Model file for the job. Use its own axes, mm. A direction names the side the tool comes from. Coordinates: 2 decimals unless noted, no trailing zeros. Order: outer loops, then holes, each group sorted by start corner. A loop starts at its lowest first (then second) coordinate and runs counter-clockwise, first axis right, second up.
from build123d import *

# Parameters (mm, degrees)
BOSS_EXTRUDE1_DEPTH = 52
SKETCH4_W           = 4
SKETCH4_H           = 10
CUT_EXTRUDE1_DEPTH  = 6
SKETCH5_W           = 4
SKETCH5_H           = 10
CUT_EXTRUDE2_DEPTH  = 6
CUT_EXTRUDE3_DEPTH  = 3
CUT_EXTRUDE4_DEPTH  = 3
SKETCH8_R           = 1
CUT_EXTRUDE5_DEPTH  = 10
SKETCH9_R           = 1
CUT_EXTRUDE6_DEPTH  = 10


with BuildPart() as part:
    # Sketch1 → Boss-Extrude1 (new body)
    with BuildSketch(Plane.XY):
        Polygon((-37.100108605, 13.346711561), (-47.100108605, 3.346711561), (-32.100108605, 3.346711561), (-32.100108605, 13.346711561), align=None)
    extrude(amount=BOSS_EXTRUDE1_DEPTH)

    # Sketch4 → Cut-Extrude1 (cut)
    with BuildSketch(Plane.XY.offset(52)):
        with Locations((-34.100108605, 8.346711561)):
            Rectangle(SKETCH4_W, SKETCH4_H)
    extrude(amount=-CUT_EXTRUDE1_DEPTH, mode=Mode.SUBTRACT)

    # Sketch5 → Cut-Extrude2 (cut)
    with BuildSketch(Plane(origin=(0, 0, 0), x_dir=(-1, 0, 0), z_dir=(0, 0, -1))):
        with Locations((34.100108605, 8.346711561)):
            Rectangle(SKETCH5_W, SKETCH5_H)
    extrude(amount=-CUT_EXTRUDE2_DEPTH, mode=Mode.SUBTRACT)

    # Sketch6 → Cut-Extrude3 (cut)
    with BuildSketch(Plane.XY.offset(52)):
        Polygon((-47.100108605, 3.346711561), (-37.100108605, 13.346711561), (-36.100108605, 13.346711561), (-36.100108605, 3.346711561), align=None)
    extrude(amount=-CUT_EXTRUDE3_DEPTH, mode=Mode.SUBTRACT)

    # Sketch7 → Cut-Extrude4 (cut)
    with BuildSketch(Plane(origin=(0, 0, 0), x_dir=(-1, 0, 0), z_dir=(0, 0, -1))):
        Polygon((47.100108605, 3.346711561), (37.100108605, 13.346711561), (36.100108605, 13.346711561), (36.100108605, 3.346711561), align=None)
    extrude(amount=-CUT_EXTRUDE4_DEPTH, mode=Mode.SUBTRACT)

    # Sketch8 → Cut-Extrude5 (cut)
    with BuildSketch(Plane(origin=(0, 0, 6), x_dir=(-1, 0, 0), z_dir=(0, 0, -1))):
        with Locations((34.100108605, 8.346711561)):
            Circle(SKETCH8_R)
    extrude(amount=-CUT_EXTRUDE5_DEPTH, mode=Mode.SUBTRACT)

    # Sketch9 → Cut-Extrude6 (cut)
    with BuildSketch(Plane.XY.offset(46)):
        with Locations((-34.100108605, 8.346711561)):
            Circle(SKETCH9_R)
    extrude(amount=-CUT_EXTRUDE6_DEPTH, mode=Mode.SUBTRACT)


solid = part.part
Q1. Cut at A-A, the plane y = 12.5. List the corners of the cut face in (x, z), plus the area to 3 significant figures.
Established:
outline: (-37.95, 3) - (-36.1, 3) - (-36.1, 6) - (-32.1, 6) - (-32.1, 46) - (-36.1, 46) - (-36.1, 49) - (-37.95, 49) - close
area: 245 mm2
Q2. Probe line 1 (Z direction, x = -36, y = 9); line 2 (X direction, y = 8, z = 14); line 3 (Y direction, x = -42.75, z = 15.5). List the from-to ranges inside material, lowest first.
Established:
line 1: z = 6 to 46
line 2: x = -42.45 to -35.04, -33.16 to -32.1
line 3: y = 3.35 to 7.7
Q3. Drop flat-ended pins along their axis: P1, Ø1.5, axis at y = 10, z = 5, coming from the +X side; P2, Ø4, axis at x = -45.5, z = 44, coming from the +Y side; P3, Ø1.5, axis at x = -43.5, z = 27, coming from the +Y side; P4, Ø4, axis at x = -43.5, y = 11, coming from the -Z side. Give the stop position or say it passes through.
Established:
P1: stops at x = -36.1
P2: stops at y = 6.95
P3: stops at y = 7.7
P4: passes through
Q4. Which spindle directions (+Z, -Z, +X, -X, +Y, -Y) get a long thin tool onto all of the face, cutting with end or side? Do faces 1 (the face through (-34, 8, 16)), 2 (the face through (-36.1, 8, 4)), 3 (the face through (-34, 10, 46)). Say none if no direction does.
Established:
face 1: -Z
face 2: -Z, +X, +Y, -Y
face 3: +Z, +X, +Y, -Y
Q5. Cut at C-C, the plane x = -34.25. List the corners of the cut face in (y, z).
Established:
outline: (3.35, 6) - (7.36, 6) - (7.36, 16) - (9.34, 16) - (9.34, 6) - (13.35, 6) - (13.35, 46) - (9.34, 46) - (9.34, 36) - (7.36, 36) - (7.36, 46) - (3.35, 46) - close
Q6. Cut at D-D, the plane z = 21.5. List the corners of the cut face in (x, y).
Established:
outline: (-47.1, 3.35) - (-32.1, 3.35) - (-32.1, 13.35) - (-37.1, 13.35) - close
Q7. Cut at B-B, the plane z = 39.5. List the corners of the cut face in (x, y).
Established:
outline: (-47.1, 3.35) - (-32.1, 3.35) - (-32.1, 13.35) - (-37.1, 13.35) - close; hole circle Ø2 at (-34.1, 8.35)
Q8. Mould opens along X. For faces 4 (the face through (-34, 10, 6)), 5 (the face through (-36.1, 8, 48)), 6 (the face through (-34, 8, 36)) say: pulls with the +X half, pulls with the -X half, needs draft (parallel to the pull), parting line crosses it, or undercut.
Established:
face 4: needs draft
face 5: pulls with the +X half
face 6: undercut
